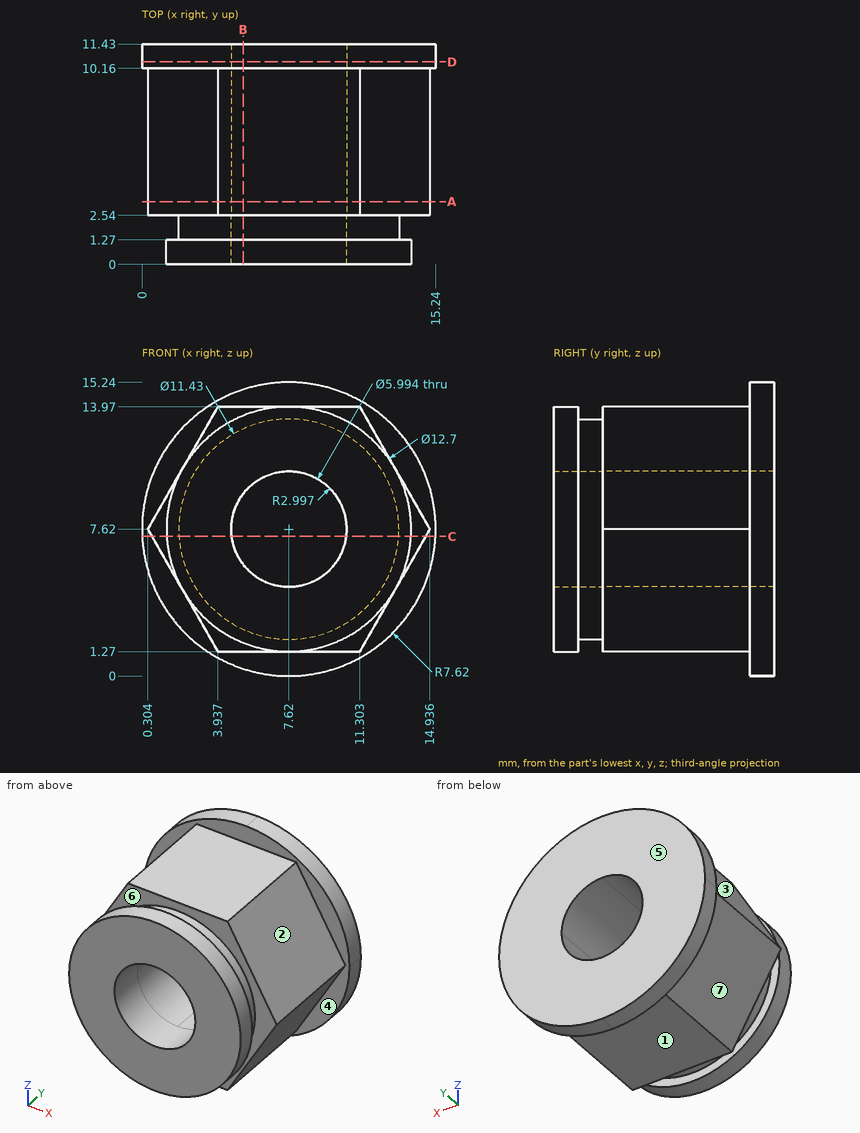
Check sheet for the drawn part. Datum: minimum x, y, z corner. Units: mm. A direction names the side the tool comes from. Round coordinates to 2 decimals unless told otherwise and drop trailing zeros. Loops run counter-clockwise (first coordinate to the right, second up) from the corner with the lowest first, then second, coordinate; pieces in that order, holes last. Notation, with made-up numbers: (14, -28.5) -> (52, -28.5) arc R17 ccw to (52, -2.5) -> close; hole circle Ø3 at (-23.75, 59). An arc over 180 degrees is marked (long way). Put each result on its own line as item: value. Start each with the question number.
1. Scan lines: probe 1 along Z at (x, y) = (7.62, 1.95) (1 decimal); probe 2 along Y at (x, z) = (3, 13.5); probe 3 along Y at (x, z) = (10.5, 1.75). Record each from-to range of solid material in increasing order.
2. Section check D-D (y = 10.5). Enter the section's corners in (x, z) (1 decimal), plus the area to 3 significant figures.
3. Gauge pin test, flat ends, axial feed: pin 1 (2 mm diameter, centred on y = 9, z = 5.5, fed in from -X) (1 decimal); pin 2 (8 mm diameter, centred on x = 7.62, z = 7.62, fed in from -Y); pin 3 (3 mm diameter, centred on x = 11.5, y = 8, fed in from +Z); pin 4 (6 mm diameter, centred on x = 8.5, y = 4.5, fed in from -Z). Record the tip position at first contact, or that the pin passes through.
4. Access from +Z, -Z, +X, -X, +Y, -Y to the whole of each face (thin tool, end or side, straight path). Record for the marked faces 1, 2 and 3.
5. Draft check along Y on the marked faces 4, 5, 6 and 7. Enter one of: +Y half, -Y half, draft (parallel to the pull), parting line (faces both ways), or undercut.
6. Section check B-B (x = 5.25). Enter the section's corners in (y, z) (1 decimal).
7. Section check A-A (y = 3.25). Enter the section's corners in (x, z) (1 decimal).
8. Section check C-C (z = 7.25). Enter the section's corners in (x, y) (1 decimal).
Findings:
1. probe 1: z = 1.9 to 4.6, 10.6 to 13.3
1. probe 2: y = 10.16 to 11.43
1. probe 3: y = 2.54 to 11.43
2. outline: (0, 7.6) arc R7.6 ccw to (7.6, 0) arc R7.6 ccw to (15.2, 7.6) arc R7.6 ccw to (7.6, 15.2) arc R7.6 ccw to start; hole (4.6, 7.6) arc R3 ccw to (7.6, 4.6) arc R3 ccw to (10.6, 7.6) arc R3 ccw to (7.6, 10.6) arc R3 ccw to start
2. area: 154 mm^2
3. pin 1: stops at x = 0.9
3. pin 2: stops at y = 0
3. pin 3: stops at z = 13.97
3. pin 4: stops at z = 1.27
4. face 1: -Z, +X, -X, -Y
4. face 2: +Z, +X, -Y
4. face 3: +Z, -X, -Y
5. face 4: -Y half
5. face 5: +Y half
5. face 6: undercut
5. face 7: draft
6. outline: (0, 1.7) -> (1.3, 1.7) -> (1.3, 2.4) -> (2.5, 2.4) -> (2.5, 1.3) -> (10.2, 1.3) -> (10.2, 0.4) -> (11.4, 0.4) -> (11.4, 5.8) -> (0, 5.8) -> close; (0, 9.5) -> (11.4, 9.5) -> (11.4, 14.9) -> (10.2, 14.9) -> (10.2, 14) -> (2.5, 14) -> (2.5, 12.8) -> (1.3, 12.8) -> (1.3, 13.5) -> (0, 13.5) -> close
7. outline: (0.3, 7.6) -> (3.9, 1.3) -> (11.3, 1.3) -> (14.9, 7.6) -> (11.3, 14) -> (3.9, 14) -> close; hole (4.6, 7.6) arc R3 ccw to (7.6, 4.6) arc R3 ccw to (10.6, 7.6) arc R3 ccw to (7.6, 10.6) arc R3 ccw to start
8. outline: (0, 10.2) -> (0.5, 10.2) -> (0.5, 2.5) -> (1.9, 2.5) -> (1.9, 1.3) -> (1.3, 1.3) -> (1.3, 0) -> (4.6, 0) -> (4.6, 11.4) -> (0, 11.4) -> close; (10.6, 0) -> (14, 0) -> (14, 1.3) -> (13.3, 1.3) -> (13.3, 2.5) -> (14.7, 2.5) -> (14.7, 10.2) -> (15.2, 10.2) -> (15.2, 11.4) -> (10.6, 11.4) -> close
